Verification items for this drawing (mm, ordinates from the low corner). A direction names the side the tool comes from. Round coordinates to 2 decimals unless told otherwise and drop trailing zeros. Write each loop counter-clockwise with the first axis right and the second up, starting at its lowest first coordinate (ties: lowest second). Pieces come first, ordered by that corner, then holes. Notation, with made-up numbers: (78.25, 31) -> (121.25, 31) arc R15 ccw to (121.25, 41) -> close; hole circle Ø4 at (79.25, 70.25). An arc over 180 degrees is marked (long way). One line per item, written item: value.
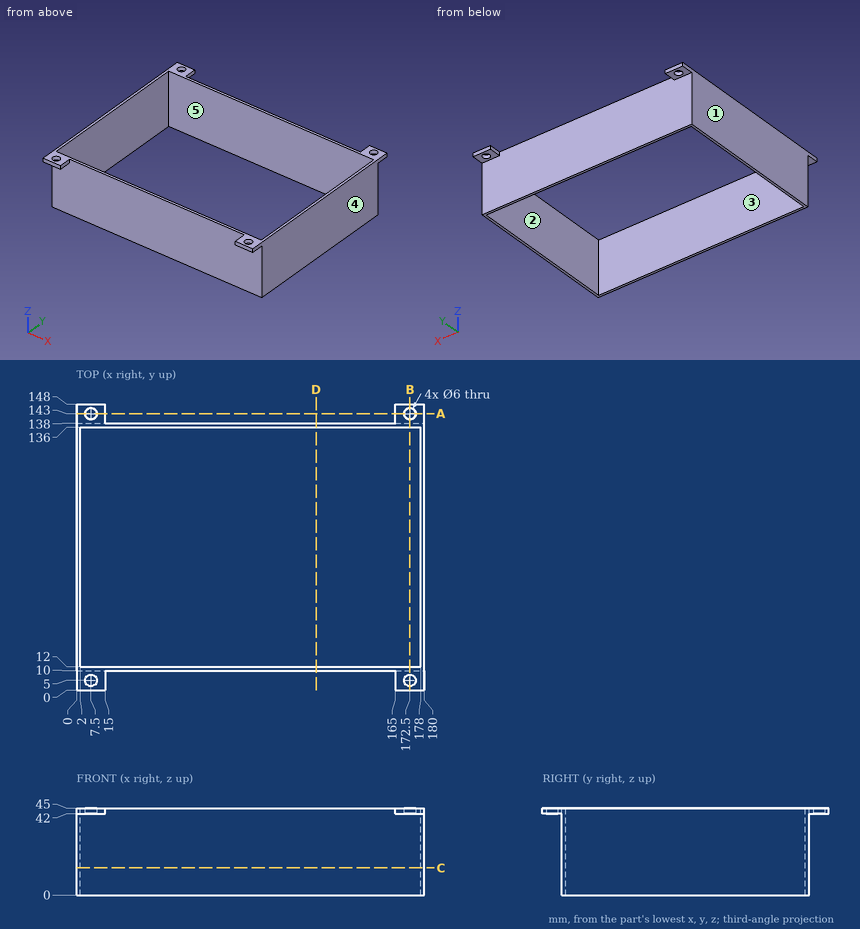
Item 1: Tool access check on the marked faces 1 and 2. Record the directions out of +Z, -Z, +X, -X, +Y, -Y that give a thin tool (end or side, any length) a straight path to the whole face; none if there is none.
Result set:
face 1: +Z, -Z, -X, +Y, -Y
face 2: +Z, -Z
Item 2: Sectioned sample at A-A (y = 143). Enter the section's corners in (x, z), then the cut area to 3 significant figures.
Result set:
outline: (0, 42) -> (4.5, 42) -> (4.5, 45) -> (0, 45) -> close; (10.5, 42) -> (15, 42) -> (15, 45) -> (10.5, 45) -> close; (165, 42) -> (169.5, 42) -> (169.5, 45) -> (165, 45) -> close; (175.5, 42) -> (180, 42) -> (180, 45) -> (175.5, 45) -> close
area: 54.0 mm^2
Item 3: Material ranges on line 1 along Y through (x, z) = (172.5, 43.2); line 2 along X through (y, z) = (143, 43); line 3 along Y through (x, z) = (24.5, 27), recorded low to high.
Result set:
line 1: 0 to 2, 8 to 12, 136 to 140, 146 to 148
line 2: 0 to 4.5, 10.5 to 15, 165 to 169.5, 175.5 to 180
line 3: 10 to 12, 136 to 138
Item 4: Release check for a two-part mould opening along Y. For the marked faces 3, 4 and 5 record: pulls with the +Y half, pulls with the -Y half, needs draft (parallel to the pull), parting line crosses it, or undercut.
Result set:
face 3: undercut
face 4: needs draft
face 5: undercut
Item 5: Sectioned sample at C-C (z = 14). Enter the section's corners in (x, y).
Result set:
outline: (0, 10) -> (180, 10) -> (180, 138) -> (0, 138) -> close; hole (2, 12) -> (178, 12) -> (178, 136) -> (2, 136) -> close
Item 6: Sectioned sample at D-D (x = 124). Enter the section's corners in (y, z).
Result set:
outline: (10, 0) -> (12, 0) -> (12, 45) -> (10, 45) -> close; (136, 0) -> (138, 0) -> (138, 45) -> (136, 45) -> close
Item 7: Depth check by flat-ended pin: pin 1 (5 mm diameter, centred on x = 10.5, y = 143, fed in from -Z); pin 2 (3 mm diameter, centred on x = 21.5, z = 20, fed in from -Y); pin 3 (1.5 mm diameter, centred on x = 64.5, z = 7, fed in from +Y); pin 4 (3.5 mm diameter, centred on x = 7.5, y = 5, fed in from -Z). Enter the tip coordinate at first touch or a pass-through.
Result set:
pin 1: z = 42
pin 2: y = 10
pin 3: y = 138
pin 4: through
Item 8: Sectioned sample at B-B (x = 172.5). Enter the section's corners in (y, z), then the cut area to 3 significant figures.
Result set:
outline: (0, 42) -> (2, 42) -> (2, 45) -> (0, 45) -> close; (8, 42) -> (10, 42) -> (10, 0) -> (12, 0) -> (12, 45) -> (8, 45) -> close; (136, 0) -> (138, 0) -> (138, 42) -> (140, 42) -> (140, 45) -> (136, 45) -> close; (146, 42) -> (148, 42) -> (148, 45) -> (146, 45) -> close
area: 204 mm^2
